Check sheet for the drawn part. Datum: minimum x, y, z corner. Units: mm. Give positions to 0.01 mm unless a question says otherwise; leave off trailing zeros. Write each loop counter-clockwise with the first axis right and the second up, starting at its lowest first coordinate (ties: lowest second). Pieces come first, ordered by that corner, then holes. Notation, with made-up numbers: (-36.5, -18) - (5.5, -18) arc R27 ccw to (5.5, 3) - close; hole circle Ø8 at (75, -26.75). An arc over 180 degrees is marked (long way). One line per question, with ' | ' between items. Start each with the question number.
Q1. Section check C-C on x = 14.5. Record the boundary of the cut face in (y, z), and give its area (3 significant figures).
Q2. Gauge pin test, flat ends, axial feed: P1, Ø24, axis at x = 25, z = 26, coming from the -Y side; P2, Ø1, axis at x = 13.5, y = 2, coming from the +Z side; P3, Ø2, axis at x = 30.5, y = 1.5, coming from the -Z side. Record the tip position at first contact, or that the pin passes through.
Q3. Release check for a two-part mould opening along X. For the marked faces 1, 2, 3 and 4 record: +X half, -X half, draft (parallel to the pull), parting line (faces both ways), or undercut.
Q4. Thickness scan on L1, parallel to Z at x = 22.5, y = 1.95; L2, parallel to X at y = 6.2, z = 22.5; L3, parallel to Z at x = 22.5, y = 3.25. Record the ranges inside material, lowest first. Write a range as [from, to].
Q5. Section check B-B on y = 1. Record the boundary of the cut face in (x, z), and give its area (3 significant figures).
Q6. Section check A-A on z = 22.5. Record the boundary of the cut face in (x, y).
Q7. Section check D-D on z = 29. Record the boundary of the cut face in (x, y).
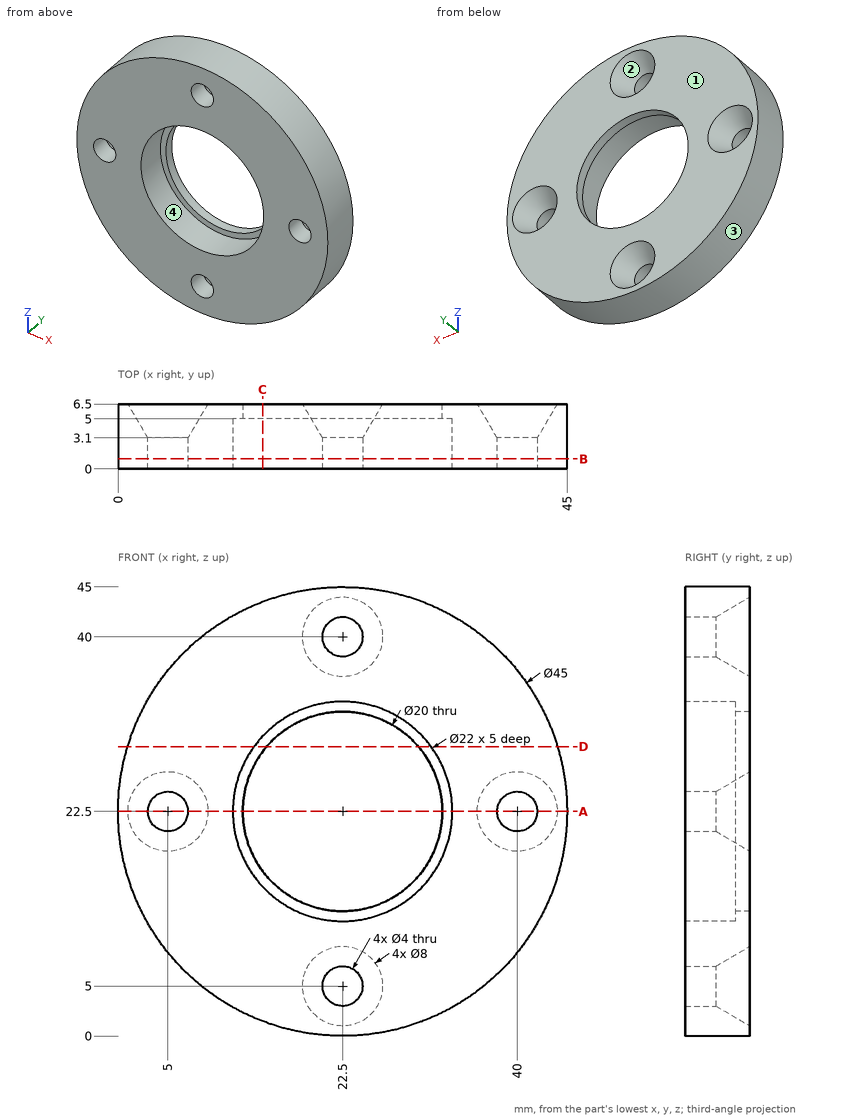
Working result:
1) outline: (0, 1.47) - (6.5, 1.47) - (6.5, 16.5) - (5, 16.5) - (5, 14.95) - (0, 14.95) - close; (0, 30.05) - (5, 30.05) - (5, 28.5) - (6.5, 28.5) - (6.5, 43.53) - (0, 43.53) - close | area: 180 mm2
2) P1: stops at y = 0 | P2: stops at z = 43.33 | P3: stops at z = 1.12
3) face 1: draft | face 2: undercut | face 3: parting line | face 4: undercut
4) L1: z = [0, 3], [7, 11.5], [33.5, 38], [42, 45] | L2: x = [0, 1.18], [8.82, 12.5], [32.5, 36.18], [43.82, 45] | L3: z = [0, 2.91], [7.09, 11.5], [33.5, 37.91], [42.09, 45]
5) outline: circle Ø45 at (22.5, 22.5); hole circle Ø4 at (5, 22.5); hole circle Ø22 at (22.5, 22.5); hole circle Ø4 at (22.5, 5); hole circle Ø4 at (22.5, 40); hole circle Ø4 at (40, 22.5) | area: 1,160 mm2
6) outline: (0, 0) - (3, 0) - (3, 3.1) - (1, 6.5) - (0, 6.5) - close; (7, 0) - (11.5, 0) - (11.5, 5) - (12.5, 5) - (12.5, 6.5) - (9, 6.5) - (7, 3.1) - close; (32.5, 5) - (33.5, 5) - (33.5, 0) - (38, 0) - (38, 3.1) - (36, 6.5) - (32.5, 6.5) - close; (42, 0) - (45, 0) - (45, 6.5) - (44, 6.5) - (42, 3.1) - close
7) outline: (0.96, 0) - (13.63, 0) - (13.63, 5) - (14.9, 5) - (14.9, 6.5) - (0.96, 6.5) - close; (30.1, 5) - (31.37, 5) - (31.37, 0) - (44.04, 0) - (44.04, 6.5) - (30.1, 6.5) - close
